from build123d import *

# Parameters (mm, degrees)
F0_W     = 77.161081
F0_H     = 76.441064
F0_W_2   = 76.700576
F0_H_2   = 58.707238
F0_H_3   = 9.812578
F1_DEPTH = 25.4
F2_DEPTH = 25.4
F3_DEPTH = 25.4


with BuildPart() as f1:
    # F0 (on Right) → F1 (new body)
    with BuildSketch(Plane.YZ):
        with Locations((38.58054, 38.220532)):
            Rectangle(F0_W, F0_H)
        Polygon((0, -74.503794), (0, 0), (0, 76.441064), (-76.700576, 76.441064), (-76.700576, -74.503794), align=None)
        Polygon((77.161081, 0), (0, 0), (0, -74.503794), (0, -75.962201), (77.161081, -75.962201), align=None)
        Polygon((155.054316, 0), (77.161081, 0), (77.161081, -75.962201), (77.161081, -76.639667), (155.054316, -76.639667), align=None)
        with Locations((-38.350288, 105.794683)):
            Rectangle(F0_W_2, F0_H_2)
        with Locations((-38.350288, 140.054591)):
            Rectangle(F0_W_2, F0_H_3)
    extrude(amount=F1_DEPTH)

    # F1_face (on face) → F2 (join)
    with BuildSketch(Plane(origin=(25.4, 14.503292, 10.620267), x_dir=(0, 1, 0), z_dir=(1, 0, 0))):
        Polygon((62.657789, 65.820798), (-14.503292, 65.820798), (-14.503292, 134.340613), (-91.203867, 134.340613), (-91.203867, -85.124061), (-14.503292, -85.124061), (-14.503292, -86.582468), (62.657789, -86.582468), (62.657789, -87.259934), (140.551024, -87.259934), (140.551024, -10.620267), (62.657789, -10.620267), align=None)
    extrude(amount=-F2_DEPTH)

    # F1_face (on face) → F3 (join)
    with BuildSketch(Plane(origin=(25.4, 14.503292, 10.620267), x_dir=(0, 1, 0), z_dir=(1, 0, 0))):
        Polygon((62.657789, 65.820798), (-14.503292, 65.820798), (-14.503292, 134.340613), (-91.203867, 134.340613), (-91.203867, -85.124061), (-14.503292, -85.124061), (-14.503292, -86.582468), (62.657789, -86.582468), (62.657789, -87.259934), (140.551024, -87.259934), (140.551024, -10.620267), (62.657789, -10.620267), align=None)
    extrude(amount=F3_DEPTH)


solid = f1.part
Input: part model. Units: mm. Frame: model coordinates. A direction names the side the tool comes from. Coordinates: 2 decimals unless noted, no trailing zeros. Loops run counter-clockwise (first coordinate to the right, second up) from the corner with the lowest first, then second, coordinate; pieces in that order, holes last.
Q1. Cut plane A-A (x = 10.5). Output: boundary loops of the cut face in (y, z), then the cut area to 3 significant figures.
Q2. Material intervals for line 1 (Z direction, x = 43, y = 45.5); line 2 (Y direction, x = 20.5, z = 35.5); line 3 (Z direction, x = 34, y = -25.5), sorted ascending.
Q3. Cut plane C-C (y = 89). Output: boundary loops of the cut face in (x, z).
Q4. Contact query for flat-ended pins moving along their axis: pin 1 (0.7 mm diameter, centred on x = 25, z = -75.5, fed in from -Y); pin 2 (3 mm diameter, centred on x = 7.5, z = 19.5, fed in from +Y). Output: stop coordinate, or through.
Q5. Set-up query: faces 1 (the face through (38, -76.701, 37)), 2 (the face through (25, 0, 110)), 3 (the face through (25, -39, -74.504)). Return all of +Z, -Z, +X, -X, +Y, -Y with unobstructed straight access to the full face (end or side cutting, diameter ignored); none if empty.
Working result:
1. outline: (-76.7, -74.5) - (0, -74.5) - (0, -75.96) - (77.16, -75.96) - (77.16, -76.64) - (155.05, -76.64) - (155.05, 0) - (77.16, 0) - (77.16, 76.44) - (0, 76.44) - (0, 144.96) - (-76.7, 144.96) - close
1. area: 34,600 mm2
2. line 1: z = -75.96 to 76.44
2. line 2: y = -76.7 to 77.16
2. line 3: z = -74.5 to 144.96
3. outline: (0, -76.64) - (50.8, -76.64) - (50.8, 0) - (0, 0) - close
4. pin 1: stops at y = 0
4. pin 2: stops at y = 77.16
5. face 1: +Z, -Z, +X, -X, -Y
5. face 2: +Z, +X, -X, +Y
5. face 3: -Z, +X, -X, -Y
